Autodesk Inventor part; units mm, degrees
ref_plane "YZ Plane" through (0, 0, 0) normal (1, 0, 0) x (0, 1, 0)
ref_plane "XZ Plane" through (0, 0, 0) normal (0, 1, 0) x (-1, 0, 0)
ref_plane "XY Plane" through (0, 0, 0) normal (0, 0, 1) x (1, 0, 0)
sketch "Sketch1" plane through (0, 0, 0) normal (0, 1, 0) x (-1, 0, 0)
  line L0 (0, 0) -> (90, 0) construction
  line L1 (90, 0) -> (90, 175)
  line L2 (90, 175) -> (0, 175)
  line L3 (0, 175) -> (0, 0) construction
  line L4 (90, 125) -> (0, 125)
  line L5 (0, 125) -> (0, 75) construction
  line L6 (0, 75) -> (90, 75)
  line L7 (90, 75) -> (90, 125)
  line L8 (30, 125) -> (30, 75)
  line L9 (27.5, 75) -> (62.5, 75) construction
  line L10 (62.5, 75) -> (62.5, 125) construction
  line L11 (62.5, 125) -> (27.5, 125) construction
  line L12 (27.5, 125) -> (27.5, 75) construction
  line L13 (27.5, 75) -> (62.5, 125) construction
  line L14 (62.5, 75) -> (27.5, 125) construction
  line L15 (90, 0) -> (90, -175)
  line L16 (90, -175) -> (0, -175)
  line L17 (90, -125) -> (0, -125)
  line L18 (0, -75) -> (90, -75)
  line L19 (90, -75) -> (90, -125)
  line L20 (30, -125) -> (30, -75)
  line L21 (27.5, -75) -> (62.5, -75) construction
  line L22 (62.5, -75) -> (62.5, -125) construction
  line L23 (62.5, -125) -> (27.5, -125) construction
  line L24 (27.5, -125) -> (27.5, -75) construction
  line L25 (27.5, -75) -> (62.5, -125) construction
  line L26 (62.5, -75) -> (27.5, -125) construction
  line L27 (-90, 0) -> (-90, 175)
  line L28 (-90, 175) -> (0, 175)
  line L29 (-90, 125) -> (0, 125)
  line L30 (0, 75) -> (-90, 75)
  line L31 (-90, 75) -> (-90, 125)
  line L32 (-30, 125) -> (-30, 75)
  line L33 (-27.5, 75) -> (-62.5, 75) construction
  line L34 (-62.5, 75) -> (-62.5, 125) construction
  line L35 (-62.5, 125) -> (-27.5, 125) construction
  line L36 (-27.5, 125) -> (-27.5, 75) construction
  line L37 (-27.5, 75) -> (-62.5, 125) construction
  line L38 (-62.5, 75) -> (-27.5, 125) construction
  line L39 (-90, 0) -> (-90, -175)
  line L40 (-90, -175) -> (0, -175)
  line L41 (-90, -125) -> (0, -125)
  line L42 (0, -75) -> (-90, -75)
  line L43 (-90, -75) -> (-90, -125)
  line L44 (-30, -125) -> (-30, -75)
  line L45 (-27.5, -75) -> (-62.5, -75) construction
  line L46 (-62.5, -75) -> (-62.5, -125) construction
  line L47 (-62.5, -125) -> (-27.5, -125) construction
  line L48 (-27.5, -125) -> (-27.5, -75) construction
  line L49 (-27.5, -75) -> (-62.5, -125) construction
  line L50 (-62.5, -75) -> (-27.5, -125) construction
  line L51 (45, 100) -> (90, 100) construction
  point P0 (45, -100)
  point P1 (-45, 100)
  point P2 (-45, -100)
  point P3 (45, -100)
  point P4 (-45, 100)
  dimension "d0" = 200
  dimension "d1" = 35
  dimension "d2" = 50
  dimension "d3" = 90
  dimension "d4" = 180
  dimension "d5" = 50
  dimension "d6" = 50
  dimension "d7" = 60
extrude "Extrusion1" add sketch "Sketch1" along normal blind 220 contours L15 L18 L42 L39 L27 L30 L6 L1 | L4 L29 L27 L28 L2 L1 | L6 L30 L32 L29 L4 L8 | L15 L16 L40 L39 L41 L17 | L20 L17 L41 L44 L42 L18
extrude "Extrusion2" add sketch "Sketch1" along normal blind 120 contours L6 L8 L4 L1 | L15 L17 L20 L18 | L30 L27 L29 L32 | L44 L41 L39 L42
hole "Hole1" at (-62.5, 0, 125) at (-27.5, 0, 125) at (-27.5, 0, 75) at (-62.5, 0, 75) at (-62.5, 0, -75) at (-27.5, 0, -75) at (-27.5, 0, -125) at (-62.5, 0, -125) at (62.5, 0, 75) at (27.5, 0, 75) at (27.5, 0, 125) at (62.5, 0, 125) at (62.5, 0, -125) at (27.5, 0, -125) at (27.5, 0, -75) at (62.5, 0, -75) direction (0, 1, 0) diameter 8 depth 15
fillet "Fillet1" radius 5 6 edges at (0, 220, -175) (-90, 110, -175) (90, 110, -175) (-90, 110, 175) (0, 220, 175) (90, 110, 175)
fillet "Fillet2" radius 8 24 edges at (-60, 220, -125) (-90, 170, -125) (-60, 220, -75) (-90, 170, -75) (-90, 120, -100) (-30, 220, -100) (-60, 220, 75) (-30, 220, 100) (-60, 220, 125) (-90, 170, 75) (-90, 120, 100) (-90, 170, 125) (60, 220, -75) (30, 220, -100) (60, 220, -125) (60, 220, 75) (30, 220, 100) (60, 220, 125) (90, 170, 75) (90, 170, 125) (90, 120, 100) (90, 170, -75) (90, 120, -100) (90, 170, -125)
sketch "Sketch2" plane through (0, 220, 0) normal (0, 1, 0) x (1, 0, 0)
  line L0 (90, -170) -> (-90, -170)
  circle A0 centre (0, -170) radius 5
  point P0 (0, 0)
  dimension "d21" = 10
extrude "Extrusion3" add sketch "Sketch2" along normal mid plane 10
properties part number "SACMI DPA C-RAIL BOTTOM SUPPORT"
Geometry check sheet. Reference: the model listing, model coordinates, mm. A direction names the side the tool comes from. Coordinates: 2 decimals unless noted, no trailing zeros. Order: outer loops, then holes, each group sorted by start corner. A loop starts at its lowest first (then second) coordinate and runs counter-clockwise, first axis right, second up. Notation, with made-up numbers: (-30, 36) - (29, 36) arc R35 cw to (29, 69) - close; hole circle Ø6 at (1.5, -10). An arc over 180 degrees is marked (long way). Answer as a JSON object with one key per item and string values. Group by question number.
Item 1: Draft check along X on faces 5 (the face through (-0.651, 222.152, 174.957)), 6 (the face through (-58.595, 7.605, -124.133)), 7 (the face through (-58.595, 7.605, 125.867)), 8 (the face through (1, 106, 175)). Enter one of: +X half, -X half, draft (parallel to the pull), parting line (faces both ways), or undercut.
Item 2: Sectioned sample at D-D, the plane z = -10. Record the cut outline in (x, y), and give its area (3 significant figures).
Item 3: Tool access check on faces 1 (the face through (56.476, 217.719, 72.594)), 2 (the face through (-87.719, 117.594, -100.462)), 3 (the face through (-30.2, 7.6, 77.95)), 4 (the face through (0, 225, 170)). Record the directions out of +Z, -Z, +X, -X, +Y, -Y that give a thin tool (end or side, any length) a straight path to the whole face; none if there is none.
Item 4: Depth check by flat-ended pin: pin 1 Ø8 at (x, z) = (37, -21.5) entering from +Y; pin 2 Ø10.5 at (x, z) = (-62.5, 125) entering from -Y; pin 3 Ø13 at (x, z) = (62.5, 125) entering from +Y; pin 4 Ø7 at (x, z) = (-62.5, -75) entering from +Y. Enter the tip coordinate at first touch or a pass-through.
Item 5: Scan lines: probe 1 along Z at (x, y) = (-27, 4); probe 2 along Z at (x, y) = (62, 161.5); probe 3 along X at (y, z) = (4, -125). Record each from-to range of solid material in increasing order.
Item 6: Sectioned sample at A-A, the plane z = 100. Record the cut outline in (x, y), and give its area (3 significant figures).
Item 7: Sectioned sample at C-C, the plane x = 42.5. Record the cut outline in (y, z), and give its area (3 significant figures).
Resolved:
{
 "1": {"face 5": "parting line", "face 6": "undercut", "face 7": "undercut", "face 8": "draft"},
 "2": {"outline": "(-90, 0) - (90, 0) - (90, 220) - (-90, 220) - close", "area": "39,600 mm^2"},
 "3": {"face 1": "+X, +Y", "face 2": "-X, +Y", "face 3": "-Y", "face 4": "+Z, -Z, +X, -X, +Y"},
 "4": {"pin 1": "y = 220", "pin 2": "y = 0", "pin 3": "y = 219.86", "pin 4": "y = 218.61"},
 "5": {"probe 1": "-175 to -128.97, -121.03 to -78.97, -71.03 to 71.03, 78.97 to 121.03, 128.97 to 175", "probe 2": "-175 to -125, -75 to 75, 125 to 175", "probe 3": "-90 to -66.5, -58.5 to -31.5, -23.5 to 23.5, 31.5 to 58.5, 66.5 to 90"},
 "6": {"outline": "(-90, 0) - (90, 0) - (90, 112) arc R8 ccw to (82, 120) - (30, 120) - (30, 212) arc R8 ccw to (22, 220) - (-22, 220) arc R8 ccw to (-30, 212) - (-30, 120) - (-82, 120) arc R8 ccw to (-90, 112) - close", "area": "27,500 mm^2"},
 "7": {"outline": "(0, -175) - (215, -175) arc R5 ccw to (220, -170) - (220, -133) arc R8 ccw to (212, -125) - (120, -125) - (120, -75) - (212, -75) arc R8 ccw to (220, -67) - (220, 67) arc R8 ccw to (212, 75) - (120, 75) - (120, 125) - (212, 125) arc R8 ccw to (220, 133) - (220, 170) arc R5 ccw to (215, 175) - (0, 175) - close", "area": "66,900 mm^2"}
}
